Autodesk Inventor part; units mm, degrees
ref_plane "YZ Plane" through (0, 0, 0) normal (1, 0, 0) x (0, 1, 0)
ref_plane "XZ Plane" through (0, 0, 0) normal (0, 1, 0) x (-1, 0, 0)
ref_plane "XY Plane" through (0, 0, 0) normal (0, 0, 1) x (1, 0, 0)
sketch "Sketch1" plane through (0, 0, 0) normal (0, 0, 1) x (1, 0, 0)
  line L0 (-160, 110) -> (-60, 0)
  line L1 (-60, 0) -> (60, 0)
  line L2 (60, 0) -> (160, 110)
  line L3 (160, 110) -> (-160, 110)
  point P0 (0, 0)
  point P1 (0, 0)
  point P2 (0, 110)
  dimension "d0" = 110
  dimension "d1" = 120
  dimension "d2" = 320
extrude "Plate1" add sketch "Sketch1" along normal blind 2
fillet "Corner Round1" radius 2 2 edges at (160, 110, 1) (-160, 110, 1)
equation "\"d3\" = Thickness"
equation "\"BendRadius\" = Thickness"
equation "\"BendReliefWidth\" = Thickness"
equation "\"BendReliefDepth\" = 0.5 * Thickness"
equation "\"CornerReliefSize\" = 4 * Thickness"
equation "\"MinimumRemnant\" = 2 * Thickness"
equation "\"TransitionRadius\" = BendRadius"
equation "\"JacobiRadiusSize\" = BendRadius"
equation "\"GapSize\" = Thickness"
properties part number "ДМФ 052 торец лотка кормовой v2.0"
Geometry: final body of the model. Coordinates: model frame, mm. Round coordinates to 2 decimals unless told otherwise and drop trailing zeros. Loops run counter-clockwise (first coordinate to the right, second up) from the corner with the lowest first, then second, coordinate; pieces in that order, holes last.
Q1. Section B-B on x = 68. Return loops of the section in (y, z).
Q2. Pin query (flat end, axial travel): P1, Ø10, axis at x = -71.5, y = 14.5, coming from the -Z side. Return the tip coordinate at first contact, or that it passes through.
Q3. Material intervals for L1, parallel to X at y = 59.5, z = 0.25; L2, parallel to Y at x = 96, z = 1.7; L3, parallel to X at y = 20, z = 0.9, sorted ascending.
Q4. Section A-A on z = 1.3. Return loops of the section in (x, y).
Q5. Section C-C on y = 88. Return loops of the section in (x, z).
Evaluation:
1. outline: (8.8, 0) - (110, 0) - (110, 2) - (8.8, 2) - close
2. P1: stops at z = 0
3. L1: x = -114.09 to 114.09
3. L2: y = 39.6 to 110
3. L3: x = -78.18 to 78.18
4. outline: (-156.96, 106.65) - (-60, 0) - (60, 0) - (156.96, 106.65) arc R2 ccw to (155.48, 110) - (-155.48, 110) arc R2 ccw to start
5. outline: (-140, 0) - (140, 0) - (140, 2) - (-140, 2) - close
